The model under review builds one solid part; all positions refer to its coordinate system, in mm. Face numbers are marked on the shaded views. A direction names the side the tool comes from. Round coordinates to 2 decimals unless told otherwise and drop trailing zeros. Order: outer loops, then holes, each group sorted by start corner. A loop starts at its lowest first (then second) coordinate and runs counter-clockwise, first axis right, second up. Notation, with made-up numbers: (-20, 65.5) -> (6, 65.5) arc R20 ccw to (6, 70.5) -> close; hole circle Ø1 at (1, 70.25). An arc over 180 degrees is marked (long way). Use a Markdown table: item, result. Add a question column.
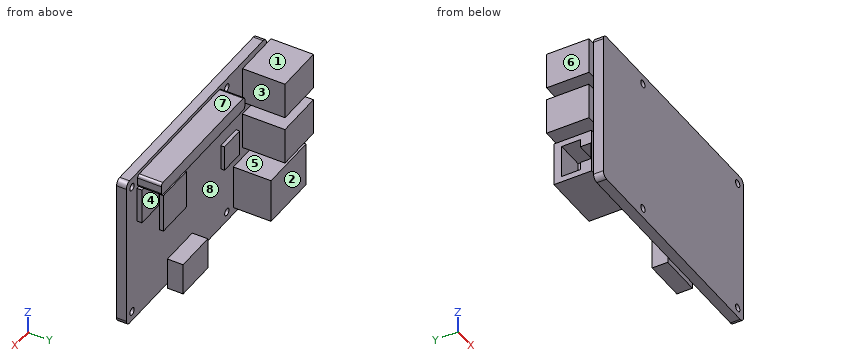
```python
from build123d import *

# Parameters (mm, degrees)
SKETCH1_R           = 1.3
BOSS_EXTRUDE1_DEPTH = 3.5
SKETCH1_3_W         = 21.23
SKETCH1_3_H         = 16
BOSS_EXTRUDE2_DEPTH = 13.5
SKETCH1_4_W         = 2.76
SKETCH1_4_H         = 13.2
SKETCH1_4_W_2       = 14.5
BOSS_EXTRUDE3_DEPTH = 15.25
SKETCH1_5_W         = 14
SKETCH1_5_H         = 14
BOSS_EXTRUDE4_DEPTH = 1.5
SKETCH1_6_W         = 15
SKETCH1_6_H         = 11.5
BOSS_EXTRUDE5_DEPTH = 5.6
SKETCH1_7_W         = 9.2
SKETCH1_7_H         = 9.2
BOSS_EXTRUDE6_DEPTH = 1.35
SKETCH1_8_W         = 10.45
SKETCH1_8_H         = 12.9
BOSS_EXTRUDE7_DEPTH = 1.8
BOSS_EXTRUDE8_DEPTH = 8.5
CUT_EXTRUDE1_DEPTH  = 10


with BuildPart() as part:
    # Sketch1 → Boss-Extrude1 (new body)
    with BuildSketch(Plane(origin=(0, 0, 0), x_dir=(1, 0, 0), z_dir=(0, 1, 0))):
        with BuildLine():
            Line((2, 0), (83, 0))
            ThreePointArc((83, 0), (84.414213562, 0.585786438), (85, 2))
            Line((85, 2), (85, 54))
            ThreePointArc((85, 54), (84.414213562, 55.414213562), (83, 56))
            Line((83, 56), (2, 56))
            ThreePointArc((2, 56), (0.585786438, 55.414213562), (0, 54))
            Line((0, 54), (0, 2))
            ThreePointArc((0, 2), (0.585786438, 0.585786438), (2, 0))
        make_face()
        with Locations(Location((81.5, 52.5, 0), (0, 0, 270))):
            Circle(SKETCH1_R, mode=Mode.SUBTRACT)
        with Locations(Location((81.5, 3.5, 0), (0, 0, 270))):
            Circle(SKETCH1_R, mode=Mode.SUBTRACT)
        with Locations(Location((24, 52.5, 0), (0, 0, 270))):
            Circle(SKETCH1_R, mode=Mode.SUBTRACT)
        with Locations(Location((24, 3.5, 0), (0, 0, 270))):
            Circle(SKETCH1_R, mode=Mode.SUBTRACT)
    extrude(amount=-BOSS_EXTRUDE1_DEPTH)

    # Sketch1_3 → Boss-Extrude2 (add)
    with BuildSketch(Plane(origin=(0, 0, 0), x_dir=(1, 0, 0), z_dir=(0, 1, 0))):
        with Locations((9.385, 45.5)):
            Rectangle(SKETCH1_3_W, SKETCH1_3_H)
    extrude(amount=BOSS_EXTRUDE2_DEPTH)

    # Sketch1_4 → Boss-Extrude3 (add)
    with BuildSketch(Plane(origin=(0, 0, 0), x_dir=(1, 0, 0), z_dir=(0, 1, 0))):
        with Locations((-1.38, 26.98)):
            Rectangle(SKETCH1_4_W, SKETCH1_4_H)
        with Locations((7.25, 26.98)):
            Rectangle(SKETCH1_4_W_2, SKETCH1_4_H)
        with Locations((-1.38, 9.1)):
            Rectangle(SKETCH1_4_W, SKETCH1_4_H)
        with Locations((7.25, 9.1)):
            Rectangle(SKETCH1_4_W_2, SKETCH1_4_H)
    extrude(amount=BOSS_EXTRUDE3_DEPTH)

    # Sketch1_5 → Boss-Extrude4 (add)
    with BuildSketch(Plane(origin=(0, 0, 0), x_dir=(1, 0, 0), z_dir=(0, 1, 0))):
        with Locations((58, 24.5)):
            Rectangle(SKETCH1_5_W, SKETCH1_5_H)
    extrude(amount=BOSS_EXTRUDE4_DEPTH)

    # Sketch1_6 → Boss-Extrude5 (add)
    with BuildSketch(Plane(origin=(0, 0, 0), x_dir=(1, 0, 0), z_dir=(0, 1, 0))):
        with Locations((52.5, 52.25)):
            Rectangle(SKETCH1_6_W, SKETCH1_6_H)
    extrude(amount=BOSS_EXTRUDE5_DEPTH)

    # Sketch1_7 → Boss-Extrude6 (add)
    with BuildSketch(Plane(origin=(0, 0, 0), x_dir=(1, 0, 0), z_dir=(0, 1, 0))):
        with Locations((23.1, 28.4)):
            Rectangle(SKETCH1_7_W, SKETCH1_7_H)
    extrude(amount=BOSS_EXTRUDE6_DEPTH)

    # Sketch1_8 → Boss-Extrude7 (add)
    with BuildSketch(Plane(origin=(0, 0, 0), x_dir=(1, 0, 0), z_dir=(0, 1, 0))):
        with Locations((73.275, 12.468354001)):
            Rectangle(SKETCH1_8_W, SKETCH1_8_H)
    extrude(amount=BOSS_EXTRUDE7_DEPTH)

    # Sketch1_9 → Boss-Extrude8 (add)
    with BuildSketch(Plane(origin=(0, 0, 0), x_dir=(1, 0, 0), z_dir=(0, 1, 0))):
        with BuildLine():
            Line((27.5, 2.25), (27.5, 4.918354001))
            ThreePointArc((27.5, 4.918354001), (27.792893219, 5.625460782), (28.5, 5.918354001))
            Line((28.5, 5.918354001), (77.1, 5.918354001))
            ThreePointArc((77.1, 5.918354001), (77.807106781, 5.625460782), (78.1, 4.918354001))
            Line((78.1, 4.918354001), (78.1, 2.25))
            ThreePointArc((78.1, 2.25), (77.807106781, 1.542893219), (77.1, 1.25))
            Line((77.1, 1.25), (28.5, 1.25))
            ThreePointArc((28.5, 1.25), (27.792893219, 1.542893219), (27.5, 2.25))
        make_face()
    extrude(amount=BOSS_EXTRUDE8_DEPTH)

    # Sketch3 → Cut-Extrude1 (cut)
    with BuildSketch(Plane.ZY.offset(1.23)):
        Polygon((-51.4, 10.7), (-39.6, 10.7), (-39.6, 4.03), (-42.41, 4.03), (-42.41, 0.23), (-48.59, 0.23), (-48.59, 4.03), (-51.4, 4.03), align=None)
    extrude(amount=-CUT_EXTRUDE1_DEPTH, mode=Mode.SUBTRACT)


solid = part.part
```
Q1. Add section C-C, the plane y = 6.5. Give the boundary of the cut face in (x, z).
Q2. Add section D-D, the plane x = 81.5. Give the boundary of the cut face in (y, z).
Q3. For pin 1 (12 mm diameter, centred on x = 59.5, z = -15, fed in from +Y); pin 2 (1 mm diameter, centred on y = 6, z = -10.5, fed in from +X); pin 3 (6 mm diameter, centred on y = 2.5, z = -55, fed in from -X), all flat-tipped, find the tip position at first contact; note any pin that passes through.
Q4. Draft analysis for pull direction X (two halves, no side actions). For the marked faces 6, 7 and 8, state which applies: released by +X, released by -X, zero draft, split by the parting line, or undercut.
Q5. For the marked faces 1, 2, 3, 4 and 5, list the 3-axis set-ups (+Z, -Z, +X, -X, +Y, -Y) from which the entire face can be reached by the end or side of a thin tool; tool diameter is ignored.
Q6. Add section B-B, the plane z = -52.5. Give the boundary of the cut face in (x, y), then the cut area to 3 significant figures.
Q7. Add section A-A, the plane x = 24. Give the boundary of the cut face in (y, z).
Q8. To check wall thickness, follow line 1 along X through (y, z) = (-1.55, -3.5); line 2 along Z through (x, y) = (81.5, -1.2); line 3 along Y through (x, z) = (59, -12.5). State the ranges of each line that lie inside material, in increasing order.
Return value:
| question | item | result |
|---|---|---|
| 1 | outline | (-2.76, -33.58) -> (14.5, -33.58) -> (14.5, -20.38) -> (-2.76, -20.38) -> close; (-2.76, -15.7) -> (14.5, -15.7) -> (14.5, -2.5) -> (-2.76, -2.5) -> close; (-1.23, -53.5) -> (20, -53.5) -> (20, -37.5) -> (-1.23, -37.5) -> (-1.23, -39.6) -> (8.77, -39.6) -> (8.77, -51.4) -> (-1.23, -51.4) -> close; (27.5, -4.92) arc R1 ccw to (28.5, -5.92) -> (77.1, -5.92) arc R1 ccw to (78.1, -4.92) -> (78.1, -2.25) arc R1 ccw to (77.1, -1.25) -> (28.5, -1.25) arc R1 ccw to (27.5, -2.25) -> close |
| 2 | outline | (-3.5, -56) -> (0, -56) -> (0, -53.8) -> (-3.5, -53.8) -> close; (-3.5, -51.2) -> (0, -51.2) -> (0, -4.8) -> (-3.5, -4.8) -> close; (-3.5, -2.2) -> (0, -2.2) -> (0, 0) -> (-3.5, 0) -> close |
| 3 | pin 1 | y = 1.5 |
| 3 | pin 2 | x = 14.5 |
| 3 | pin 3 | x = -1.23 |
| 4 | face 6 | released by -X |
| 4 | face 7 | zero draft |
| 4 | face 8 | undercut |
| 5 | face 1 | +Z, -X, +Y |
| 5 | face 2 | -Z, +X, -X, +Y |
| 5 | face 3 | +Z, +Y |
| 5 | face 4 | -Z, +X, +Y |
| 5 | face 5 | +X, -X, +Y |
| 6 | outline | (-1.23, 0) -> (0, 0) -> (0, -3.5) -> (22.7, -3.5) -> (22.7, 0) -> (20, 0) -> (20, 13.5) -> (-1.23, 13.5) -> close; (25.3, -3.5) -> (80.2, -3.5) -> (80.2, 0) -> (60, 0) -> (60, 5.6) -> (45, 5.6) -> (45, 0) -> (25.3, 0) -> close; (82.8, -3.5) -> (85, -3.5) -> (85, 0) -> (82.8, 0) -> close |
| 6 | area | 650 mm² |
| 7 | outline | (-3.5, -56) -> (0, -56) -> (0, -53.8) -> (-3.5, -53.8) -> close; (-3.5, -51.2) -> (0, -51.2) -> (0, -33) -> (1.35, -33) -> (1.35, -23.8) -> (0, -23.8) -> (0, -4.8) -> (-3.5, -4.8) -> close; (-3.5, -2.2) -> (0, -2.2) -> (0, 0) -> (-3.5, 0) -> close |
| 8 | line 1 | 0 to 22.7, 25.3 to 80.2, 82.8 to 85 |
| 8 | line 2 | -56 to -53.8, -51.2 to -4.8, -2.2 to 0 |
| 8 | line 3 | -3.5 to 0 |
